Part model, mm, in its own coordinate system. Face numbers are marked on the shaded views. Round coordinates to 2 decimals unless told otherwise and drop trailing zeros. Loops run counter-clockwise (first coordinate to the right, second up) from the corner with the lowest first, then second, coordinate; pieces in that order, holes last.
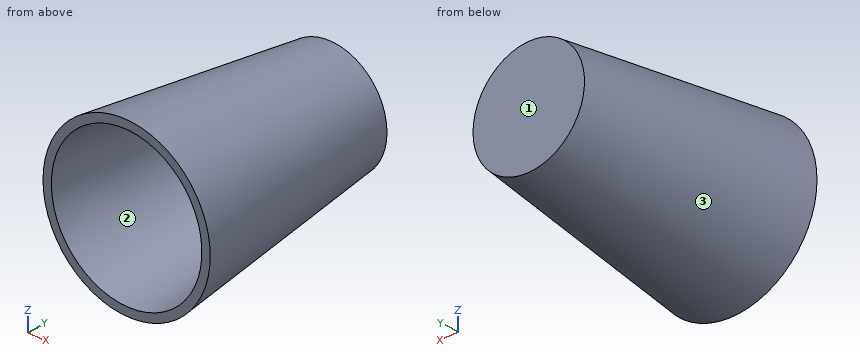
from build123d import *

# Parameters (mm, degrees)
F0_R     = 25.4
F2_R     = 38.1
F5_R     = 21.59
F4_R     = 34.29
F7_R     = 24.9738959908
F8_DEPTH = 2.54


with BuildPart() as f3:
    # F0 (on Front) → F3 section 0
    with BuildSketch(Plane.XZ):
        Circle(F0_R)
    # F2 (on offset) → F3 section 1
    with BuildSketch(Plane.XZ.offset(101.6)):
        Circle(F2_R)
    loft()

    # F5 (on face) → F6 section 0
    with BuildSketch(Plane(origin=(0, 0, 0), x_dir=(-1, 0, 0), z_dir=(0, 1, 0))):
        Circle(F5_R)
    # F4 (on face) → F6 section 1
    with BuildSketch(Plane.XZ.offset(101.6)):
        Circle(F4_R)
    loft(mode=Mode.SUBTRACT)

    # F7 (on Front) → F8 (join)
    with BuildSketch(Plane.XZ):
        Circle(F7_R)
    extrude(amount=F8_DEPTH)


solid = f3.part
1) Slice it at B-B, the plane y = -44.5. Give the cut face in (x, z) (1 decimal).
Values:
outline: circle Ø61.9 at (0, 0); hole circle Ø54.3 at (0, 0)
2) Slice it at C-C, the plane y = -69.5. Give the cut face in (x, z) (1 decimal), then the cut area to 3 significant figures.
Values:
outline: circle Ø68.2 at (0, 0); hole circle Ø60.6 at (0, 0)
area: 770 mm2
3) Wall check: line 1 along Z through (x, y) = (20, -59.5); line 2 along Y through (x, z) = (9.5, -8); line 3 along Z through (x, y) = (5.5, -27). Give the ranges that are in metal, low to high.
Values:
line 1: z = -26.04 to -21.04, 21.04 to 26.04
line 2: y = -2.54 to 0
line 3: z = -28.24 to -24.35, 24.35 to 28.24
4) Slice it at A-A, the plane x = 0. Give the cut face in (y, z), then the cut area to 3 significant figures.
Values:
outline: (-101.6, -38.1) - (0, -25.4) - (0, 25.4) - (-101.6, 38.1) - (-101.6, 34.29) - (-2.54, 21.91) - (-2.54, -21.91) - (-101.6, -34.29) - close
area: 885 mm2
5) Drop flat-ended pins along their axis: pin 1 Ø8 at (y, z) = (-46.5, 6.5) entering from -X; pin 2 Ø4 at (y, z) = (-57, -13) entering from -X; pin 3 Ø8 at (y, z) = (-25.5, -30.5) entering from -X. Give the stop position or say it passes through.
Values:
pin 1: stops at x = -31.35
pin 2: stops at x = -30.66
pin 3: stops at x = -10.81
6) Mould opens along X. For the marked faces 1, 2 and 3 say: released by +X, released by -X, zero draft, split by the parting line, or undercut.
Values:
face 1: zero draft
face 2: undercut
face 3: split by the parting line
